from build123d import *

# Parameters (mm, degrees)
F1_DEPTH = 57.5
F2_T     = -2
F3_R     = 4
F4_DEPTH = 25


with BuildPart() as f1:
    # F0 (on Front) → F1 (new body, symmetric)
    with BuildSketch(Plane.XZ):
        with BuildLine():
            Line((17.5, 7.8446282016), (17.5, 9.6824583655))
            ThreePointArc((17.5, 9.6824583655), (-20, 0), (17.5, -9.6824583655))
            Line((17.5, -9.6824583655), (17.5, -7.8446282016))
            Line((17.5, -7.8446282016), (22.5, -7.8446282016))
            Line((22.5, -7.8446282016), (22.5, 7.8446282016))
            Line((22.5, 7.8446282016), (17.5, 7.8446282016))
        make_face()
    extrude(amount=F1_DEPTH, both=True)

    # F2
    f2_openings = [f1.faces().sort_by_distance(p)[0] for p in [
        (0.740007, 57.5, 0),
    ]]
    offset(amount=F2_T, openings=f2_openings, kind=Kind.INTERSECTION)

    # F3 (on face) → F4 (cut)
    with BuildSketch(Plane.XZ.offset(57.5)):
        Circle(F3_R)
    extrude(amount=-F4_DEPTH, mode=Mode.SUBTRACT)


solid = f1.part
Check sheet for the modelled part. Datum: model origin and axes. Units: mm. A direction names the side the tool comes from. Round coordinates to 2 decimals unless told otherwise and drop trailing zeros. Loops run counter-clockwise (first coordinate to the right, second up) from the corner with the lowest first, then second, coordinate; pieces in that order, holes last. Notation, with made-up numbers: (54, 79.5) -> (68, 79.5) arc R20 ccw to (68, 95.5) -> close; hole circle Ø7 at (-30, -25.75). An arc over 180 degrees is marked (long way). Put each result on its own line as item: value. Start each with the question number.
1. Section check D-D (x = 9). Enter the section's corners in (y, z).
2. Draft check along X on faces 1 (the face through (22.5, -1, 0)), 2 (the face through (-19.986, -0.805, 0.738)), 3 (the face through (20, -1, -7.845)), 4 (the face through (20.5, 0, 0)). Enter one of: +X half, -X half, draft (parallel to the pull), parting line (faces both ways), or undercut.
3. Section check B-B (z = 0). Enter the section's corners in (x, y), plus the area to 3 significant figures.
4. Scan lines: probe 1 along Z at (x, y) = (0, -56.6); probe 2 along Z at (x, y) = (0, 3); probe 3 along Y at (x, z) = (8, 3). Record each from-to range of solid material in increasing order.
5. Section check C-C (y = -4). Enter the section's corners in (x, z), plus the area to 3 significant figures.
6. Gauge pin test, flat ends, axial feed: pin 1 (0.6 mm diameter, centred on y = 4.5, z = -8.5, fed in from +X); pin 2 (1.5 mm diameter, centred on x = 19, y = 24.5, fed in from -Z); pin 3 (2.5 mm diameter, centred on x = 20.5, y = 21.5, fed in from +Z). Record the tip position at first contact, or that the pin passes through.
7. Access from +Z, -Z, +X, -X, +Y, -Y to the whole of each face (thin tool, end or side, straight path). Record for faces 5 (the face through (15.5, 0, -8)), 6 (the face through (17, 57.5, 6)), 7 (the face through (20, -1, 7.845)).
8. Section check A-A (x = 0). Enter the section's corners in (y, z).
Findings:
1. outline: (-57.5, -17.86) -> (57.5, -17.86) -> (57.5, -15.59) -> (-55.5, -15.59) -> (-55.5, 15.59) -> (57.5, 15.59) -> (57.5, 17.86) -> (-57.5, 17.86) -> close
2. face 1: +X half
2. face 2: parting line
2. face 3: draft
2. face 4: undercut
3. outline: (-20, -57.5) -> (-4, -57.5) -> (-4, -55.5) -> (-18, -55.5) -> (-18, 57.5) -> (-20, 57.5) -> close; (4, -57.5) -> (22.5, -57.5) -> (22.5, 57.5) -> (20.5, 57.5) -> (20.5, -55.5) -> (4, -55.5) -> close
3. area: 521 mm^2
4. probe 1: z = -20 to -4, 4 to 20
4. probe 2: z = -20 to -18, 18 to 20
4. probe 3: y = -57.5 to -55.5
5. outline: (17.5, -9.68) -> (17.5, -7.84) -> (22.5, -7.84) -> (22.5, 7.84) -> (17.5, 7.84) -> (17.5, 9.68) arc R20 ccw (long way) to start; hole (15.5, -9.15) -> (15.5, -5.84) -> (20.5, -5.84) -> (20.5, 5.84) -> (15.5, 5.84) -> (15.5, 9.15) arc R18 ccw (long way) to start
5. area: 257 mm^2
6. pin 1: stops at x = 17.5
6. pin 2: stops at z = -7.84
6. pin 3: stops at z = 7.84
7. face 5: +Y
7. face 6: +Z, -Z, +X, -X, +Y
7. face 7: +Z, +X, +Y, -Y
8. outline: (-57.5, -20) -> (57.5, -20) -> (57.5, -18) -> (-55.5, -18) -> (-55.5, -4) -> (-57.5, -4) -> close; (-57.5, 4) -> (-55.5, 4) -> (-55.5, 18) -> (57.5, 18) -> (57.5, 20) -> (-57.5, 20) -> close
